Part model, mm, in its own coordinate system. Face numbers are marked on the shaded views. A direction names the side the tool comes from. Give positions to 0.01 mm unless a question says otherwise; leave off trailing zeros. Order: outer loops, then holes, each group sorted by start corner. A loop starts at its lowest first (then second) coordinate and runs counter-clockwise, first axis right, second up. Notation, with made-up numbers: M 44.5,9.25 L 99.5,9.25 A16 ccw 99.5,37.25 Z; hole C 52.5,46 d1. An arc over 180 degrees is marked long. Write each question's results on one line, items separated by ' | '. Start each with the question number.
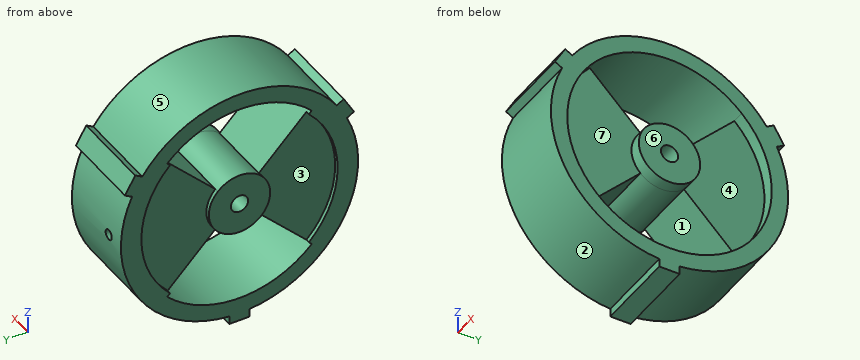
from build123d import *

# Parameters (mm, degrees)
CROQUIS2_R              = 25
CROQUIS2_R_2            = 7.5
CORTAR_EXTRUIR1_DEPTH   = 3
CORTAR_EXTRUIR3_DEPTH   = 73
CROQUIS4_R              = 1.25
CORTAR_EXTRUIR4_DEPTH   = 20
CROQUIS5_R              = 1
CORTAR_EXTRUIR5_DEPTH   = 10
CORTAR_EXTRUIR6_START   = -1
CROQUIS6_R              = 24
CROQUIS6_R_2            = 7.5
CORTAR_EXTRUIR6_DEPTH   = 1
SALIENTE_EXTRUIR1_START = -20
SALIENTE_EXTRUIR1_DEPTH = 20
MATRIZC1_COUNT          = 3


with BuildPart() as part:
    # Croquis1 → Revolución1 (revolve)
    with BuildSketch(Plane.XY, mode=Mode.PRIVATE) as revoluci_n1_sk:
        Polygon((-10, 29), (-10, 2.1), (0, 2.1), (10, 2.1), (10, 29), align=None)
    revolve(revoluci_n1_sk.sketch.rotate(Axis((0, 0, 0), (1, 0, 0)), 90), axis=Axis((0, 0, 0), (1, 0, 0)))

    # Croquis2 → Cortar-Extruir1 (cut)
    with BuildSketch(Plane(origin=(10, 0, 0), x_dir=(0, 0, -1), z_dir=(1, 0, 0))):
        Circle(CROQUIS2_R)
        Circle(CROQUIS2_R_2, mode=Mode.SUBTRACT)
    extrude(amount=-CORTAR_EXTRUIR1_DEPTH, mode=Mode.SUBTRACT)

    # Croquis3 → Cortar-Extruir3 (cut)
    with BuildSketch(Plane(origin=(10, 0, 0), x_dir=(0, 0, -1), z_dir=(1, 0, 0))):
        with BuildLine():
            ThreePointArc((-5.303301, -5.303301), (-7.5, 0), (-5.303301, 5.303301))
            Line((-5.303301, 5.303301), (-17.67767, 17.67767))
            ThreePointArc((-17.67767, 17.67767), (-25, 0), (-17.67767, -17.67767))
            Line((-17.67767, -17.67767), (-5.303301, -5.303301))
        make_face()
        with BuildLine():
            ThreePointArc((17.67767, -17.67767), (25, 0), (17.67767, 17.67767))
            Line((17.67767, 17.67767), (5.303301, 5.303301))
            ThreePointArc((5.303301, 5.303301), (7.5, 0), (5.303301, -5.303301))
            Line((5.303301, -5.303301), (17.67767, -17.67767))
        make_face()
    extrude(amount=-CORTAR_EXTRUIR3_DEPTH, mode=Mode.SUBTRACT)

    # Croquis4 → Cortar-Extruir4 (cut)
    with BuildSketch(Plane(origin=(0, 30, 0), x_dir=(1, 0, 0), z_dir=(0, 1, 0))):
        with Locations(Location((-5, 0, 0), (0, 0, 270))):
            Circle(CROQUIS4_R)
    extrude(amount=-CORTAR_EXTRUIR4_DEPTH, mode=Mode.SUBTRACT)

    # Croquis5 → Cortar-Extruir5 (cut)
    with BuildSketch(Plane(origin=(0, 10, 0), x_dir=(1, 0, 0), z_dir=(0, 1, 0))):
        with Locations(Location((-5, 0, 0), (0, 0, 270))):
            Circle(CROQUIS5_R)
    extrude(amount=-CORTAR_EXTRUIR5_DEPTH, mode=Mode.SUBTRACT)

    # Croquis6 → Cortar-Extruir6 (cut)
    with BuildSketch(Plane.ZY.offset(10).offset(CORTAR_EXTRUIR6_START)):
        Circle(CROQUIS6_R)
        with Locations(Location((0, 0, 0), (0, 0, 180))):
            Circle(CROQUIS6_R_2, mode=Mode.SUBTRACT)
    extrude(amount=CORTAR_EXTRUIR6_DEPTH, mode=Mode.SUBTRACT)

    # Croquis7 → Saliente-Extruir1 (add)
    with BuildSketch(Plane(origin=(10, 0, 0), x_dir=(0, 0, -1), z_dir=(1, 0, 0)).offset(SALIENTE_EXTRUIR1_START)):
        with BuildLine():
            Line((29, -2.5), (29, 0))
            ThreePointArc((29, 0), (28.972998, -1.251165), (28.89204, -2.5))
            Line((28.89204, -2.5), (29, -2.5))
        make_face()
        Polygon((30.89204, 2.5), (29, 2.5), (29, 0), (29, -2.5), (30.89204, -2.5), align=None)
        with BuildLine():
            Line((29, 0), (29, 2.5))
            Line((29, 2.5), (28.89204, 2.5))
            ThreePointArc((28.89204, 2.5), (28.972998, 1.251165), (29, 0))
        make_face()
    saliente_extruir1 = extrude(amount=SALIENTE_EXTRUIR1_DEPTH)

    # MatrizC1: Saliente-Extruir1 ×3 about axis
    matrizc1_axis = Axis((0, 0, 0), (1, 0, 0))
    for i in range(1, MATRIZC1_COUNT):
        add(saliente_extruir1.rotate(matrizc1_axis, i * 360 / MATRIZC1_COUNT))


solid = part.part
(1) Tool access for the marked faces 1, 2, 3 and 4: list every direction of +Z, -Z, +X, -X, +Y, -Y with a clear straight run to the whole face (end or side of a thin tool).
(2) Probe L1, parallel to Z at x = -5, y = 17; L2, parallel to X at y = 4, z = 0; L3, parallel to Z at x = -4.25, y = -9. List the from-to ranges inside material, lowest first.
(3) Pull direction Z, two halves, no side cores. Call the marked faces 5, 6 and 7: +Z half, -Z half, draft (parallel to the pull), parting line (faces both ways), or undercut.
(4) Saw through at D-D on y = -11. Give the cut face in (x, z), plus the area to 3 significant figures.
(5) Saw through at C-C on z = 0. Give the number of separate pieces and of enclosed holes in the cut face, plus the area to 3 significant figures.
(6) Drop flat-ended pins along their axis: P1, Ø1, axis at x = -5, y = 13, coming from the +Z side; P2, Ø2, axis at x = -2.5, z = 2.5, coming from the +Y side; P3, Ø1, axis at x = -3, y = -10.5, coming from the -Z side; P4, Ø21.5, axis at y = 18, z = -7, coming from the +X side. Give the stop position or say it passes through.
(7) Saw through at A-A on y = 13.5. Give the cut face in (x, z).
(8) Saw through at B-B on x = 5.25. Give the cut face in (y, z), plus the area to 3 significant figures.
Taken from the geometry:
1) face 1: +X, -X | face 2: +X, -X, -Y | face 3: -X | face 4: +X
2) L1: z = -23.49 to -18.33, -17 to -1.25, 1.25 to 17, 18.33 to 23.49 | L2: x = -10 to -6, -4 to 10 | L3: z = -27.57 to -23.32, -9 to 9, 23.32 to 27.57
3) face 5: +Z half | face 6: draft | face 7: undercut
4) outline: M -10,-26.83 L 10,-26.83 L 10,-22.45 L -10,-22.45 Z; M -10,22.45 L 10,22.45 L 10,26.83 L -10,26.83 Z; M -9,-11 L 7,-11 L 7,11 L -9,11 Z | area: 527 mm²
5) separate pieces: 3 | enclosed holes: 0 | area: 875 mm²
6) P1: stops at z = 26.17 | P2: stops at y = 28.96 | P3: stops at z = -27.22 | P4: stops at x = 10
7) outline: M -10,-25.67 L 10,-25.67 L 10,-21.04 L -10,-21.04 Z; M -10,21.04 L 10,21.04 L 10,25.67 L -10,25.67 Z; M -9,-13.5 L 7,-13.5 L 7,13.5 L -9,13.5 Z; hole C -5,0 d2.5
8) outline: M -28,13.28 L -26.27,12.28 A29 ccw -2.5,-28.89 L -2.5,-30.89 L 2.5,-30.89 L 2.5,-28.89 A29 ccw 26.27,12.28 L 28,13.28 L 25.5,17.61 L 23.77,16.61 A29 ccw -23.77,16.61 L -25.5,17.61 Z; hole M -17.68,-17.68 A25 ccw 17.68,-17.68 L 5.3,-5.3 A7.5 cw -5.3,-5.3 Z; hole M -17.68,17.68 L -5.3,5.3 A7.5 cw 5.3,5.3 L 17.68,17.68 A25 ccw Z; hole C 0,0 d4.2 | area: 1,760 mm²
